The listing builds one solid part. Answer for the finished solid, in the listing's coordinates (mm). Face numbers are marked on the shaded views. A direction names the side the tool comes from. Give positions to 0.01 mm unless a question says otherwise; leave off trailing zeros. Order: outer loops, then holes, each group sorted by start corner. A loop starts at its lowest first (then second) coordinate and runs counter-clockwise, first axis right, second up.
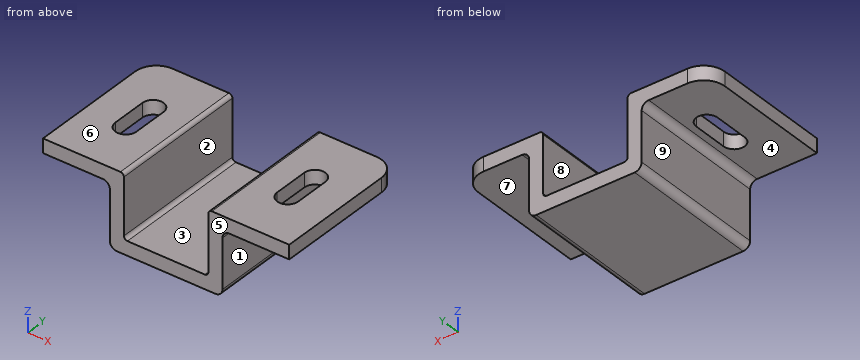
```python
from build123d import *

# Parameters (mm, degrees)
SKETCH1_W           = 35
SKETCH1_H           = 20
BOSS_EXTRUDE1_DEPTH = 2
SKETCH4_W           = 11.5
SKETCH4_H           = 20
BOSS_EXTRUDE2_DEPTH = 9
SKETCH5_W           = 9.5
SKETCH5_H           = 9
CUT_EXTRUDE2_DEPTH  = 21
FILLET1_R           = 1
FILLET2_R           = 0.5
CUT_EXTRUDE3_DEPTH  = 12
FILLET3_R           = 3


with BuildPart() as part:
    # Sketch1 → Boss-Extrude1 (new body)
    with BuildSketch(Plane.XY):
        with Locations((17.5, 10)):
            Rectangle(SKETCH1_W, SKETCH1_H)
    extrude(amount=BOSS_EXTRUDE1_DEPTH)

    # Sketch4 → Boss-Extrude2 (add)
    with BuildSketch(Plane.XY.offset(2)):
        with Locations((5.75, 10)):
            Rectangle(SKETCH4_W, SKETCH4_H)
        with Locations((29.25, 10)):
            Rectangle(SKETCH4_W, SKETCH4_H)
    extrude(amount=BOSS_EXTRUDE2_DEPTH)

    # Sketch5 → Cut-Extrude2 (cut, through all)
    with BuildSketch(Plane(origin=(0, 20, 0), x_dir=(1, 0, 0), z_dir=(0, 1, 0))):
        with Locations((4.75, -4.5)):
            Rectangle(SKETCH5_W, SKETCH5_H)
        with Locations((30.25, -4.5)):
            Rectangle(SKETCH5_W, SKETCH5_H)
    extrude(amount=-CUT_EXTRUDE2_DEPTH, mode=Mode.SUBTRACT)

    # Fillet1
    fillet1_edges = [part.edges().sort_by_distance(p)[0] for p in [
        (9.5, 10, 0),
        (9.5, 10, 9),
        (25.5, 10, 9),
        (25.5, 10, 0),
    ]]
    fillet(fillet1_edges, radius=FILLET1_R)

    # Fillet2
    fillet2_edges = [part.edges().sort_by_distance(p)[0] for p in [
        (11.5, 10, 2),
        (11.5, 10, 11),
        (23.5, 10, 2),
        (23.5, 10, 11),
    ]]
    fillet(fillet2_edges, radius=FILLET2_R)

    # Sketch2 → Cut-Extrude3 (cut, through all)
    with BuildSketch(Plane.XY.offset(11)):
        with BuildLine():
            Line((7.5, 12.5), (7.5, 7.5))
            ThreePointArc((7.5, 7.5), (6, 6), (4.5, 7.5))
            Line((4.5, 7.5), (4.5, 12.5))
            ThreePointArc((4.5, 12.5), (6, 14), (7.5, 12.5))
        make_face()
        with BuildLine():
            Line((30.5, 12.5), (30.5, 7.5))
            ThreePointArc((30.5, 7.5), (29, 6), (27.5, 7.5))
            Line((27.5, 7.5), (27.5, 12.5))
            ThreePointArc((27.5, 12.5), (29, 14), (30.5, 12.5))
        make_face()
    extrude(amount=-CUT_EXTRUDE3_DEPTH, mode=Mode.SUBTRACT)

    # Fillet3
    fillet3_edges = [part.edges().sort_by_distance(p)[0] for p in [
        (0, 20, 10),
        (35, 20, 10),
    ]]
    fillet(fillet3_edges, radius=FILLET3_R)


solid = part.part
```
1) Straight lines are drawn through the part: probe 1 along X at (y, z) = (9.5, 9.25); probe 2 along X at (y, z) = (14.5, 6.5); probe 3 along X at (y, z) = (13, 9.25). For each, find the intervals that lie inside material, in ascending order.
Geometry says:
probe 1: x = 0 to 4.5, 7.5 to 11.5, 23.5 to 27.5, 30.5 to 35
probe 2: x = 9.5 to 11.5, 23.5 to 25.5
probe 3: x = 0 to 4.59, 7.41 to 11.5, 23.5 to 27.59, 30.41 to 35
2) Given P1, Ø2.5, axis at y = 10.5, z = 8, coming from the -X side; P2, Ø5.5, axis at x = 17.5, y = 12.5, coming from the +Z side; P3, Ø9.5, axis at x = 2.5, y = 9, coming from the -Z side; P4, Ø3, axis at y = 13.5, z = 6.5, coming from the +X side, each flat-ended and moving along its own axis, determine where each tip first touches the part or whether it passes through.
Geometry says:
P1: stops at x = 0
P2: stops at z = 2
P3: stops at z = 9
P4: stops at x = 25.5
3) Find section A-A (x = 29). Write down the section's boundary in (y, z), then the cut area to 3 significant figures.
Geometry says:
outline: (0, 9) - (6, 9) - (6, 11) - (0, 11) - close; (14, 9) - (20, 9) - (20, 11) - (14, 11) - close
area: 24.0 mm2
4) A tool of negligible diameter and unlimited length cuts with its end or side. For the marked faces 5, 6, 7, 8 and 9, from which of +Z, -Z, +X, -X, +Y, -Y can it reach the whole face along a straight path? Write none if from no direction.
Geometry says:
face 5: +Z, -Z, +X, -X, -Y
face 6: +Z, +X, -X, +Y, -Y
face 7: -Z, +X, +Y, -Y
face 8: +Z, +Y, -Y
face 9: -Z, -X, +Y, -Y
5) Find section B-B (y = 9.75). Write down the section's boundary in (x, z), then the cut area to 3 significant figures.
Geometry says:
outline: (0, 9) - (4.5, 9) - (4.5, 11) - (0, 11) - close; (7.5, 9) - (8.5, 9) arc R1 cw to (9.5, 8) - (9.5, 1) arc R1 ccw to (10.5, 0) - (24.5, 0) arc R1 ccw to (25.5, 1) - (25.5, 8) arc R1 cw to (26.5, 9) - (27.5, 9) - (27.5, 11) - (24, 11) arc R0.5 ccw to (23.5, 10.5) - (23.5, 2.5) arc R0.5 cw to (23, 2) - (12, 2) arc R0.5 cw to (11.5, 2.5) - (11.5, 10.5) arc R0.5 ccw to (11, 11) - (7.5, 11) - close; (30.5, 9) - (35, 9) - (35, 11) - (30.5, 11) - close
area: 94.0 mm2
6) Find section C-C (z = 5.5). Write down the section's boundary in (x, y), then the cut area to 3 significant figures.
Geometry says:
outline: (9.5, 0) - (11.5, 0) - (11.5, 20) - (9.5, 20) - close; (23.5, 0) - (25.5, 0) - (25.5, 20) - (23.5, 20) - close
area: 80.0 mm2
7) Find section D-D (y = 4.5). Write down the section's boundary in (x, z).
Geometry says:
outline: (0, 9) - (8.5, 9) arc R1 cw to (9.5, 8) - (9.5, 1) arc R1 ccw to (10.5, 0) - (24.5, 0) arc R1 ccw to (25.5, 1) - (25.5, 8) arc R1 cw to (26.5, 9) - (35, 9) - (35, 11) - (24, 11) arc R0.5 ccw to (23.5, 10.5) - (23.5, 2.5) arc R0.5 cw to (23, 2) - (12, 2) arc R0.5 cw to (11.5, 2.5) - (11.5, 10.5) arc R0.5 ccw to (11, 11) - (0, 11) - close
8) For a pull along X with two mould halves and no side action, classify the marked faces 1, 2, 3 and 4 as +X half, -X half, draft (parallel to the pull), parting line (faces both ways), or undercut.
Geometry says:
face 1: +X half
face 2: undercut
face 3: undercut
face 4: draft
